Source: CAD feature listing. Evaluate the final solid. Frame: model axes, mm. Face numbers are marked on the shaded views. A direction names the side the tool comes from. Coordinates: 2 decimals unless noted, no trailing zeros. Order: outer loops, then holes, each group sorted by start corner. A loop starts at its lowest first (then second) coordinate and runs counter-clockwise, first axis right, second up. Notation, with made-up numbers: (-7.75, 38) -> (30.25, 38) arc R13 cw to (30.25, 53) -> close; hole circle Ø11 at (23, 77). An arc over 180 degrees is marked (long way). Write item = value, one per line. Start each with the question number.
Item 1: Ray query, line 1 along Y through (x, z) = (4.5, 2.5); line 2 along Y through (x, z) = (-2.5, -1); line 3 along Y through (x, z) = (2, 0.75). Return the intervals inside material, ascending. Write a range as [from, to].
Item 2: Section query D-D (y = 26.5). Output: boundary loops of the cut face in (x, z).
Item 3: Set-up query: the marked faces 1, 2 and 3. Return all of +Z, -Z, +X, -X, +Y, -Y with unobstructed straight access to the full face (end or side cutting, diameter ignored); none if empty.
Item 4: Section query C-C (y = 18). Output: boundary loops of the cut face in (x, z).
Item 5: Contact query for flat-ended pins moving along their axis: pin 1 (4 mm diameter, centred on x = -0.5, y = 3.5, fed in from +Z); pin 2 (3 mm diameter, centred on x = -3, y = 24, fed in from -Z); pin 3 (3 mm diameter, centred on x = -5, z = 3.5, fed in from -Y). Output: stop coordinate, or through.
Item 6: Section query B-B (x = 0). Output: boundary loops of the cut face in (y, z), then the cut area to 3 significant figures.
Item 7: Section query A-A (z = 0). Output: boundary loops of the cut face in (x, y).
Autodesk Inventor part; units mm, degrees
ref_plane "YZ Plane" through (0, 0, 0) normal (1, 0, 0) x (0, 1, 0)
ref_plane "XZ Plane" through (0, 0, 0) normal (0, 1, 0) x (-1, 0, 0)
ref_plane "XY Plane" through (0, 0, 0) normal (0, 0, 1) x (1, 0, 0)
sketch "Boceto1" plane through (0, 0, 0) normal (0, 0, 1) x (1, 0, 0)
  line L0 (0, 33) -> (-3, 33)
  line L1 (-3, 33) -> (-3, 23)
  line L2 (-3, 23) -> (-6.5, 23)
  line L3 (-6.5, 23) -> (-6.5, 15)
  line L4 (-6.5, 15) -> (-3, 15)
  line L5 (0, 0) -> (-3, 0)
  line L6 (0, 33) -> (0, 0)
  line L7 (-3, 0) -> (-3, 13)
  arc A0 (-3, 13) -> (-3, 15) centre (-3, 14) ccw
  line L8 (-3, 14) -> (-3, 13) construction
  dimension "d0" = 33
  dimension "d2" = 3
  dimension "d3" = 3
  dimension "d6" = 6.5
  dimension "d7" = 13
  dimension "d8" = 10
  dimension "d9" = 15
revolve "Revolución1" add sketch "Boceto1" angle 360 about axis through (0, 33, 0) along (0, -1, 0)
thread "Rosca1"
thread "Rosca2"
properties part number "sensor_tension"
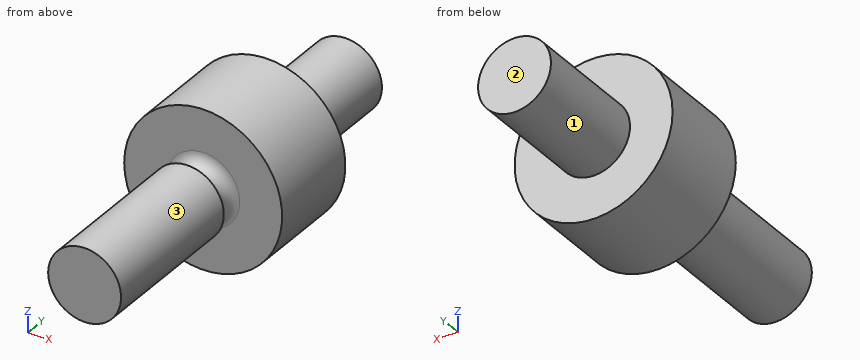
Computed:
q1.line_1 = [15, 23]
q1.line_2 = [0, 13.05], [14.95, 33]
q1.line_3 = [0, 13.5], [14.5, 33]
q2.outline = circle Ø6 at (0, 0)
q3.face_1 = +Y
q3.face_2 = +Z, -Z, +X, -X, +Y
q3.face_3 = -Y
q4.outline = circle Ø13 at (0, 0)
q5.pin_1 = 3
q5.pin_2 = -6.22
q5.pin_3 = 15
q6.outline = (0, -3) -> (13, -3) arc R1 cw to (15, -3) -> (15, -6.5) -> (23, -6.5) -> (23, -3) -> (33, -3) -> (33, 3) -> (23, 3) -> (23, 6.5) -> (15, 6.5) -> (15, 3) arc R1 cw to (13, 3) -> (0, 3) -> close
q6.area = 251 mm^2
q7.outline = (-6.5, 15) -> (-3, 15) arc R1 cw to (-3, 13) -> (-3, 0) -> (3, 0) -> (3, 13) arc R1 cw to (3, 15) -> (6.5, 15) -> (6.5, 23) -> (3, 23) -> (3, 33) -> (-3, 33) -> (-3, 23) -> (-6.5, 23) -> close
